For this review, take the finished solid that the model builds, in its own axes (mm). A direction names the side the tool comes from. Give positions to 0.01 mm unless a question says otherwise; leave off trailing zeros. Write each loop counter-clockwise with the first axis right and the second up, starting at its lowest first coordinate (ties: lowest second). Pieces come first, ordered by that corner, then holes.
from build123d import *

# Parameters (mm, degrees)
F1_DEPTH = 3


with BuildPart() as f1:
    # F0 (on Front) → F1 (new body)
    with BuildSketch(Plane.XZ):
        Polygon((-42.5, -31.6), (-42.5, -42.5), (-31.6, -42.5), (-31.6, -39.5), (-23.7, -39.5), (-23.7, -42.5), (-15.8, -42.5), (-15.8, -39.5), (-7.9, -39.5), (-7.9, -42.5), (0, -42.5), (0, -39.5), (7.9, -39.5), (7.9, -42.5), (15.8, -42.5), (15.8, -39.5), (23.7, -39.5), (23.7, -42.5), (42.5, -42.5), (42.5, -31.6), (39.5, -31.6), (39.5, -23.7), (42.5, -23.7), (42.5, -15.8), (39.5, -15.8), (39.5, -7.9), (42.5, -7.9), (42.5, 0), (42.5, 7.9), (39.5, 7.9), (39.5, 15.8), (42.5, 15.8), (42.5, 23.7), (39.5, 23.7), (39.5, 31.6), (42.5, 31.6), (42.5, 42.5), (23.7, 42.5), (23.7, 39.5), (15.8, 39.5), (15.8, 42.5), (7.9, 42.5), (7.9, 39.5), (0, 39.5), (0, 42.5), (-7.9, 42.5), (-7.9, 39.5), (-15.8, 39.5), (-15.8, 42.5), (-23.7, 42.5), (-23.7, 39.5), (-31.6, 39.5), (-31.6, 42.5), (-42.5, 42.5), (-42.5, 31.6), (-39.5, 31.6), (-39.5, 23.7), (-42.5, 23.7), (-42.5, 15.8), (-39.5, 15.8), (-39.5, 7.9), (-42.5, 7.9), (-42.5, 0), (-42.5, -7.9), (-39.5, -7.9), (-39.5, -15.8), (-42.5, -15.8), (-42.5, -23.7), (-39.5, -23.7), (-39.5, -31.6), align=None)
        with BuildLine():
            ThreePointArc((0, -30), (-30, 0), (0, 30))
            ThreePointArc((0, 30), (30, 0), (0, -30))
        make_face(mode=Mode.SUBTRACT)
    extrude(amount=F1_DEPTH)


solid = f1.part
(1) We need section A-A (z = 0). Write out the cut boundary in (x, y), and give its area (3 significant figures).
(2) Tool access review of faces 4 (the flat face through (42.5, -1, 20)), 5 (the flat face through (41, -1, -15.8)), 6 (the flat face through (-41, -1, -31.6)), 7 (the flat face through (-31.6, -1, -41)), 8 (the flat face through (-15.8, -1, 41)): name each direction out of +Z, -Z, +X, -X, +Y, -Y from which nothing blocks a thin tool from reaching the whole face with its end or side.
(3) For L1, parallel to X at y = -1.7, z = 0; L2, parallel to Z at x = 13.5, y = -2.25; L3, parallel to Z at x = 4, y = -2.4, list the stretches that pass through material, from the lowest coordinate up.
(4) The part is to be moulded in two halves that separate along Z. For faces 1 (the flat face through (-37, -1, -42.5)), 2 (the flat face through (4, -1, 39.5)), 3 (the cylindrical face through (-29.287, -1.479, -6.503)), say which applies: +Z half, -Z half, draft (parallel to the pull), parting line (faces both ways), or undercut.
(5) Clearance check with a flat-ended pin moving along its axis: pin 1 Ø1.5 at (y, z) = (-1, -14) entering from +X. State where the tip first meets the part, or that it passes through.
(6) We need section B-B (x = -3.5). Write out the cut boundary in (y, z), and give its area (3 significant figures).
The answers:
1. outline: (-42.5, -3) - (-30, -3) - (-30, 0) - (-42.5, 0) - close; (30, -3) - (42.5, -3) - (42.5, 0) - (30, 0) - close
1. area: 75.0 mm2
2. face 4: +Z, -Z, +X, +Y, -Y
2. face 5: +X, +Y, -Y
2. face 6: -X, +Y, -Y
2. face 7: -Z, +Y, -Y
2. face 8: +Z, +Y, -Y
3. L1: x = -42.5 to -30, 30 to 42.5
3. L2: z = -42.5 to -26.79, 26.79 to 42.5
3. L3: z = -39.5 to -29.73, 29.73 to 39.5
4. face 1: -Z half
4. face 2: +Z half
4. face 3: undercut
5. pin 1: stops at x = 39.5
6. outline: (-3, -42.5) - (0, -42.5) - (0, -29.8) - (-3, -29.8) - close; (-3, 29.8) - (0, 29.8) - (0, 42.5) - (-3, 42.5) - close
6. area: 76.2 mm2
